```python
from build123d import *

# Parameters (mm, degrees)
SKETCH1_W           = 140
SKETCH1_H           = 50
SKETCH1_R           = 2
BOSS_EXTRUDE1_DEPTH = 10
SKETCH2_R           = 2.5
CUT_EXTRUDE1_DEPTH  = 153


with BuildPart() as part:
    # Sketch1 → Boss-Extrude1 (new body)
    with BuildSketch(Plane.XY):
        Rectangle(SKETCH1_W, SKETCH1_H)
        with Locations((-10, 15)):
            Circle(SKETCH1_R, mode=Mode.SUBTRACT)
        with Locations(Location((10, 15, 0), (0, 0, 180))):
            Circle(SKETCH1_R, mode=Mode.SUBTRACT)
    extrude(amount=BOSS_EXTRUDE1_DEPTH)

    # Sketch2 → Cut-Extrude1 (cut)
    with BuildSketch(Plane(origin=(70, 0, 0), x_dir=(0, 0, -1), z_dir=(1, 0, 0))):
        with Locations((-5, 0)):
            Circle(SKETCH2_R)
    extrude(amount=-CUT_EXTRUDE1_DEPTH, mode=Mode.SUBTRACT)


solid = part.part
```
For this review, take the finished solid that the model builds, in its own axes (mm). Round coordinates to 2 decimals unless told otherwise and drop trailing zeros. Write each loop counter-clockwise with the first axis right and the second up, starting at its lowest first coordinate (ties: lowest second). Pieces come first, ordered by that corner, then holes. Notation, with made-up numbers: (29.25, 57) -> (58.25, 57) arc R14 ccw to (58.25, 65) -> close; hole circle Ø2 at (-32, 17). An arc over 180 degrees is marked (long way). One line per question, with ' | ' between items. Start each with the question number.
(1) Mouldability with a two-part tool opening along Y and no side actions: class faces 1 (the face through (70, 0, 2)), 2 (the face through (-1, 25, 5)), 3 (the face through (-10, 17, 5)) as released by +Y, released by -Y, zero draft, split by the parting line, or undercut.
(2) Add section C-C, the plane y = 0. Write out the cut boundary in (x, z).
(3) Insertion check: P1, Ø2.5, axis at x = 10, y = 15, coming from the -Z side. The pin has a flat end and moves straight along its axis. Give the tip position at first contact, or say it passes through.
(4) Add section A-A, the plane x = 10. Write out the cut boundary in (y, z), plus the area to 3 significant figures.
(5) For line 1 along Y through (x, z) = (10, 5.25); line 2 along X through (y, z) = (16.5, 4.5); line 3 along Y through (x, z) = (-10, 3.75), list the stretches that pass through material, from the lowest coordinate up. Write a range as from..to.
(6) Add section D-D, the plane x = 42. Write out the cut boundary in (y, z).
(7) Add section B-B, the plane z = 5. Write out the cut boundary in (x, y).
Answer list:
1) face 1: zero draft | face 2: released by +Y | face 3: undercut
2) outline: (-70, 0) -> (70, 0) -> (70, 2.5) -> (-70, 2.5) -> close; (-70, 7.5) -> (70, 7.5) -> (70, 10) -> (-70, 10) -> close
3) P1: through
4) outline: (-25, 0) -> (13, 0) -> (13, 10) -> (-25, 10) -> close; (17, 0) -> (25, 0) -> (25, 10) -> (17, 10) -> close; hole circle Ø5 at (0, 5) | area: 440 mm²
5) line 1: -25..-2.49, 2.49..13, 17..25 | line 2: -70..-11.32, -8.68..8.68, 11.32..70 | line 3: -25..-2.17, 2.17..13, 17..25
6) outline: (-25, 0) -> (25, 0) -> (25, 10) -> (-25, 10) -> close; hole circle Ø5 at (0, 5)
7) outline: (-70, -25) -> (70, -25) -> (70, -2.5) -> (-70, -2.5) -> close; (-70, 2.5) -> (70, 2.5) -> (70, 25) -> (-70, 25) -> close; hole circle Ø4 at (-10, 15); hole circle Ø4 at (10, 15)
